Source: three-view drawing plus pictorial views. Frame: mm from the lowest corner of the part. A direction names the side the tool comes from. Coordinates: 2 decimals unless noted, no trailing zeros. Write each loop counter-clockwise with the first axis right and the second up, starting at its lowest first coordinate (ties: lowest second). Pieces come first, ordered by that corner, then holes. Notation, with made-up numbers: (85.5, 22) - (129.5, 22) arc R31 cw to (129.5, 48) - close; hole circle Ø3 at (-14, 5.25). An arc over 180 degrees is marked (long way). Answer as a JSON object with one key per item and string values. Group by question number.
Item 1: Section A-A on x = 5. Return loops of the section in (y, z).
Item 2: Section C-C on y = 29. Return loops of the section in (x, z).
Item 3: Mould query, pull axis Y, two halves, no side actions, for the marked faces 3, 4 and 5. Classes: pulls with the +Y half, pulls with the -Y half, needs draft (parallel to the pull), parting line crosses it, or undercut.
Item 4: Set-up query: the marked faces 1 and 2. Return all of +Z, -Z, +X, -X, +Y, -Y with unobstructed straight access to the full face (end or side cutting, diameter ignored); none if empty.
Item 5: Line query: line 1 along Y through (x, z) = (7.75, 4.5); line 2 along X through (y, z) = (7.5, 1.5); line 3 along Z through (x, y) = (11.5, 29). Output: solid intervals per line, ascending. Write a range as from..to.
Item 6: First-contact query: pin 1 Ø1.6 at (y, z) = (16, 0.5) entering from -X; pin 2 Ø6 at (x, y) = (8.5, 20) entering from +Z; pin 3 Ø1.6 at (y, z) = (22, 0.5) entering from +X. Flat tips, straight axial feed; report the tip coordinate or a pass-through.
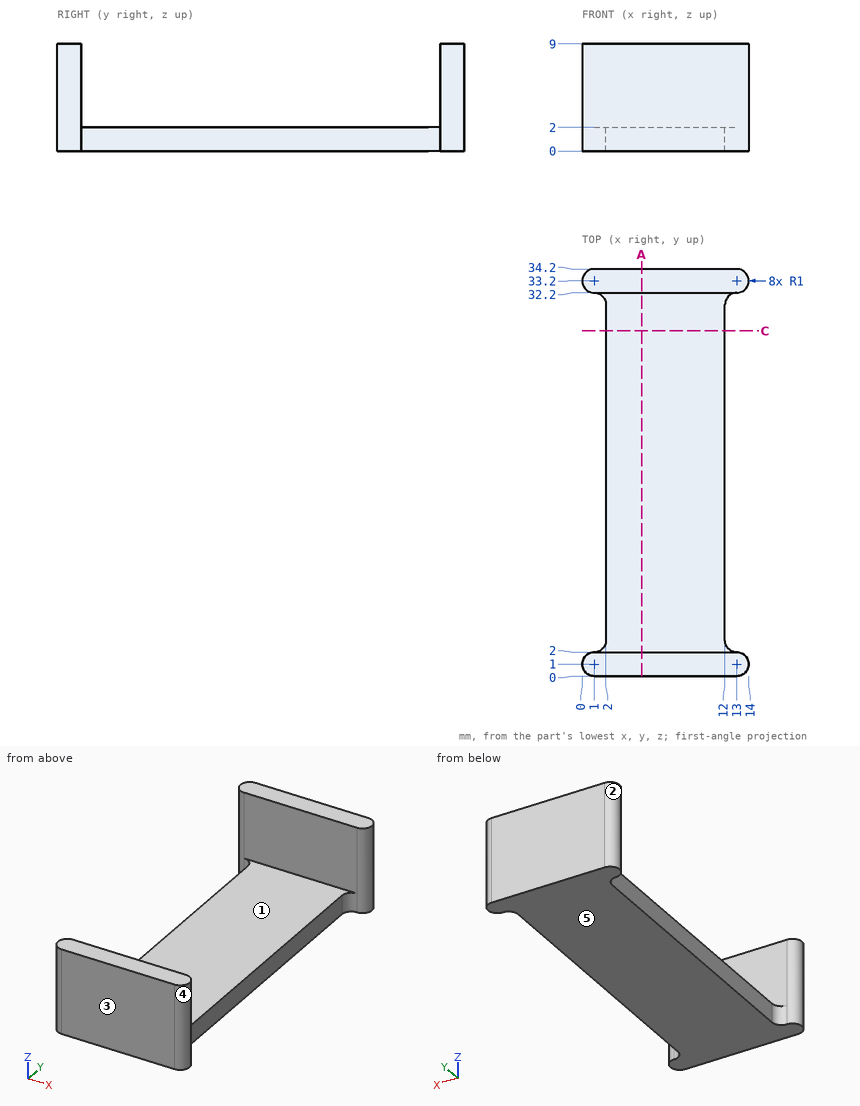
Checks:
{
 "1": {"outline": "(0, 0) - (34.2, 0) - (34.2, 9) - (32.2, 9) - (32.2, 2) - (2, 2) - (2, 9) - (0, 9) - close"},
 "2": {"outline": "(2, 0) - (12, 0) - (12, 2) - (2, 2) - close"},
 "3": {"face 3": "pulls with the -Y half", "face 4": "undercut", "face 5": "needs draft"},
 "4": {"face 1": "+Z, +X, -X", "face 2": "+Z, -Z, -X"},
 "5": {"line 1": "0..2, 32.2..34.2", "line 2": "2..12", "line 3": "0..2"},
 "6": {"pin 1": "x = 2", "pin 2": "z = 2", "pin 3": "x = 12"}
}
